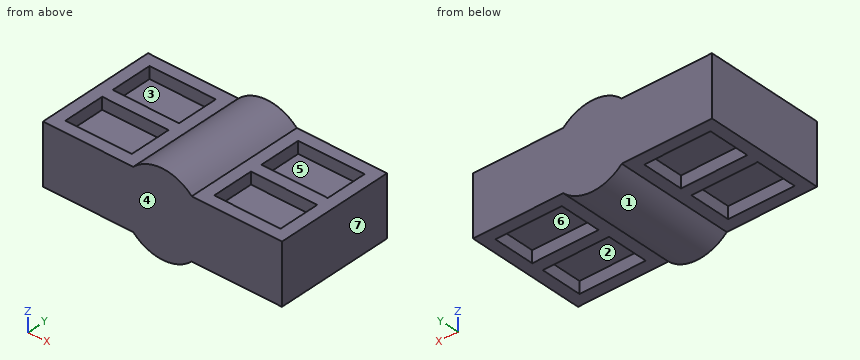
from build123d import *

# Parameters (mm, degrees)
F0_W     = 20
F0_H     = 10
F1_DEPTH = 5
F3_DEPTH = 10
F4_W     = 5.5505102572
F4_H     = 3.5
F5_DEPTH = 1
F6_W     = 5.5505102572
F6_H     = 3.5
F7_DEPTH = 1


with BuildPart() as f1:
    # F0 (on Top) → F1 (new body)
    with BuildSketch(Plane.XY):
        with Locations((10, -5)):
            Rectangle(F0_W, F0_H)
    extrude(amount=F1_DEPTH)

    # F2 (on face) → F3 (join)
    with BuildSketch(Plane.XZ.offset(10)):
        with BuildLine():
            Line((7.5505102572, 5), (12.4494897428, 5))
            ThreePointArc((12.4494897428, 5), (10, 6), (7.5505102572, 5))
        make_face()
        with BuildLine():
            ThreePointArc((7.5505102572, 0), (10, -1), (12.4494897428, 0))
            Line((12.4494897428, 0), (7.5505102572, 0))
        make_face()
    extrude(amount=-F3_DEPTH)

    # F4 (on face) → F5 (cut)
    with BuildSketch(Plane.XY.offset(5)):
        with Locations((3.7752551286, -2.75)):
            Rectangle(F4_W, F4_H)
        with Locations((3.7752551286, -7.25)):
            Rectangle(F4_W, F4_H)
        with Locations((16.2247448714, -2.75)):
            Rectangle(F4_W, F4_H)
        with Locations((16.2247448714, -7.25)):
            Rectangle(F4_W, F4_H)
    extrude(amount=-F5_DEPTH, mode=Mode.SUBTRACT)

    # F6 (on face) → F7 (cut)
    with BuildSketch(Plane(origin=(0, 0, 0), x_dir=(1, 0, 0), z_dir=(0, 0, -1))):
        with Locations((3.7752551286, 7.25)):
            Rectangle(F6_W, F6_H)
        with Locations((16.2247448714, 7.25)):
            Rectangle(F6_W, F6_H)
        with Locations((16.2247448714, 2.75)):
            Rectangle(F6_W, F6_H)
        with Locations((3.7752551286, 2.75)):
            Rectangle(F6_W, F6_H)
    extrude(amount=-F7_DEPTH, mode=Mode.SUBTRACT)


solid = f1.part
Verification items for the finished model (mm, model axes). Face numbers are marked on the shaded views. A direction names the side the tool comes from. Give positions to 0.01 mm unless a question says otherwise; leave off trailing zeros. Loops run counter-clockwise (first coordinate to the right, second up) from the corner with the lowest first, then second, coordinate; pieces in that order, holes last.
1) Draft check along X on the marked faces 4, 5, 6 and 7. Enter one of: pulls with the +X half, pulls with the -X half, needs draft (parallel to the pull), parting line crosses it, or undercut.
2) Set-up check for the marked faces 1, 2 and 3: record each of +Z, -Z, +X, -X, +Y, -Y from which the full face is reachable in a straight line by a thin tool's end or side.
3) Sectioned sample at A-A, the plane z = 4.5. Enter the section's corners in (x, y), then the cut area to 3 significant figures.
4) Sectioned sample at C-C, the plane x = 5.5. Enter the section's corners in (y, z).
5) Sectioned sample at B-B, the plane y = -4.25. Enter the section's corners in (x, z), then the cut area to 3 significant figures.
6) Thickness scan on line 1 along X through (y, z) = (-3.25, 4.5); line 2 along Y through (x, z) = (2.75, 0.75); line 3 along Z through (x, y) = (6.25, -8.5). Record the ranges inside material, lowest first.
7) Depth check by flat-ended pin: pin 1 Ø1.8 at (x, y) = (3, -7) entering from +Z; pin 2 Ø4 at (x, y) = (4, -5.5) entering from -Z; pin 3 Ø4 at (x, y) = (17.5, -7) entering from +Z. Enter the tip coordinate at first touch or a pass-through.
8) Sectioned sample at D-D, the plane y = -5.25. Enter the section's corners in (x, z), then the cut area to 3 significant figures.
Answers:
1. face 4: needs draft
1. face 5: undercut
1. face 6: undercut
1. face 7: pulls with the +X half
2. face 1: -Z, +Y, -Y
2. face 2: -Z
2. face 3: +Z
3. outline: (0, -10) - (20, -10) - (20, 0) - (0, 0) - close; hole (1, -9) - (6.55, -9) - (6.55, -5.5) - (1, -5.5) - close; hole (1, -4.5) - (6.55, -4.5) - (6.55, -1) - (1, -1) - close; hole (13.45, -9) - (19, -9) - (19, -5.5) - (13.45, -5.5) - close; hole (13.45, -4.5) - (19, -4.5) - (19, -1) - (13.45, -1) - close
3. area: 122 mm2
4. outline: (-10, 0) - (-9, 0) - (-9, 1) - (-5.5, 1) - (-5.5, 0) - (-4.5, 0) - (-4.5, 1) - (-1, 1) - (-1, 0) - (0, 0) - (0, 5) - (-1, 5) - (-1, 4) - (-4.5, 4) - (-4.5, 5) - (-5.5, 5) - (-5.5, 4) - (-9, 4) - (-9, 5) - (-10, 5) - close
5. outline: (0, 0) - (1, 0) - (1, 1) - (6.55, 1) - (6.55, 0) - (7.55, 0) arc R3.5 ccw to (12.45, 0) - (13.45, 0) - (13.45, 1) - (19, 1) - (19, 0) - (20, 0) - (20, 5) - (19, 5) - (19, 4) - (13.45, 4) - (13.45, 5) - (12.45, 5) arc R3.5 ccw to (7.55, 5) - (6.55, 5) - (6.55, 4) - (1, 4) - (1, 5) - (0, 5) - close
5. area: 84.5 mm2
6. line 1: x = 0 to 1, 6.55 to 13.45, 19 to 20
6. line 2: y = -10 to -9, -5.5 to -4.5, -1 to 0
6. line 3: z = 1 to 4
7. pin 1: stops at z = 4
7. pin 2: stops at z = 0
7. pin 3: stops at z = 5
8. outline: (0, 0) - (7.55, 0) arc R3.5 ccw to (12.45, 0) - (20, 0) - (20, 5) - (12.45, 5) arc R3.5 ccw to (7.55, 5) - (0, 5) - close
8. area: 107 mm2
